Build history of the part. All positions in model axes, mm. Face numbers are marked on the shaded views. A direction names the side the tool comes from. Give positions to 0.01 mm unless a question says otherwise; leave off trailing zeros. Write each loop counter-clockwise with the first axis right and the second up, starting at its lowest first coordinate (ties: lowest second). Pieces come first, ordered by that corner, then holes.
Autodesk Inventor part; units mm, degrees
ref_plane "Work Plane1" through (0, 16, 0) normal (0, 1, 0) x (1, 0, 0)
ref_plane "YZ Plane" through (0, 0, 0) normal (1, 0, 0) x (0, 1, 0)
ref_plane "XZ Plane" through (0, 0, 0) normal (0, 1, 0) x (-1, 0, 0)
sketch "Sketch1" plane through (0, 0, 0) normal (0, 1, 0) x (-1, 0, 0)
  circle A0 centre (0, 0) radius 1.5
  dimension "d0" = 3
extrude "Extrusion1" add sketch "Sketch1" along normal blind 14
thread "Thread1"
ref_plane "Work Plane1" through (0, 16, 0) normal (0, 1, 0) x (1, 0, 0)
sketch "Sketch4" plane through (0, 16, 0) normal (0, 1, 0) x (1, 0, 0)
  circle A0 centre (0, 0) radius 2.5
  dimension "d14" = 5
loft "Loft1" add profiles "Sketch4" section 2 edges at (1.5, 14, 0)
sketch "Sketch5" plane through (0, 16, 0) normal (0, 1, 0) x (1, 0, 0)
  circle A0 centre (0, 0) radius 2.5
  line L0 (-2.4495, 0.5) -> (2.4495, 0.5)
  line L1 (-2.4495, -0.5) -> (2.4495, -0.5)
  line L2 (0, 0) -> (2.0973, 0) construction
  dimension "d19" = 1
extrude "Extrusion4" cut sketch "Sketch5" against normal blind 1 contours A0 L1 L0
properties part number "Screw_CountersunkHead_3x16" material "Steel, Galvanized"
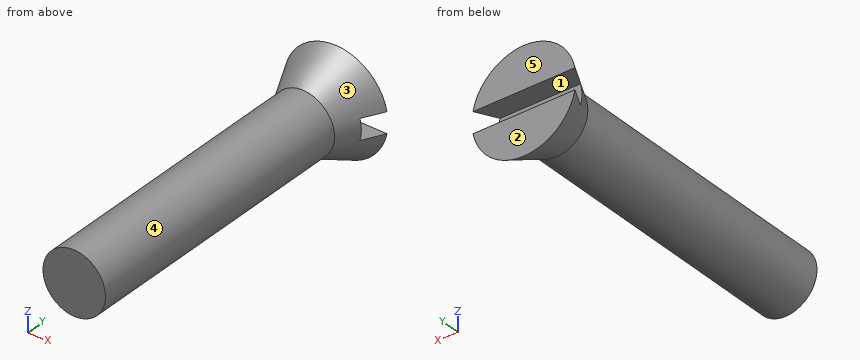
1. Saw through at B-B on y = 9.5. Give the cut face in (x, z), plus the area to 3 significant figures.
2. Mould opens along Z. For the marked faces 1, 2 and 3 say: pulls with the +Z half, pulls with the -Z half, needs draft (parallel to the pull), parting line crosses it, or undercut.
3. Saw through at A-A on x = 0. Give the cut face in (y, z), plus the area to 3 significant figures.
4. 3-axis set-ups, long thin cutter, end or side, ignore diameter. For the marked faces 4 and 5: which of +Z, -Z, +X, -X, +Y, -Y reach the whole face in a straight line?
5. Drop flat-ended pins along their axis: pin 1 (0.5 mm diameter, centred on x = 0, z = 0, fed in from +Y); pin 2 (3 mm diameter, centred on y = 9, z = 2, fed in from +X); pin 3 (1.5 mm diameter, centred on x = -1, y = 13, fed in from +Z). Give the stop position or say it passes through.
6. Drill centre lines: line 1 along Y through (x, z) = (0.9, 2.1); line 2 along X through (y, z) = (11, -0.8); line 3 along Z through (x, y) = (-0.55, 3.25). Where is each one in solid material? Low to high.
Outcome:
1. outline: circle Ø3 at (0, 0)
1. area: 7.07 mm2
2. face 1: undercut
2. face 2: needs draft
2. face 3: parting line crosses it
3. outline: (0, -1.5) - (14, -1.5) - (16, -2.5) - (16, -0.5) - (15, -0.5) - (15, 0.5) - (16, 0.5) - (16, 2.5) - (14, 1.5) - (0, 1.5) - close
3. area: 49.0 mm2
4. face 4: -Y
4. face 5: +Z, -Z, +X, -X, +Y
5. pin 1: stops at y = 15
5. pin 2: stops at x = 1.41
5. pin 3: stops at z = 1.48
6. line 1: y = 15.57 to 16
6. line 2: x = -1.27 to 1.27
6. line 3: z = -1.4 to 1.4
